Geometry check sheet. Reference: the model listing, model coordinates, mm. A direction names the side the tool comes from. Round coordinates to 2 decimals unless told otherwise and drop trailing zeros. Order: outer loops, then holes, each group sorted by start corner. A loop starts at its lowest first (then second) coordinate and runs counter-clockwise, first axis right, second up.
(1) Cross-section at C-C on x = -1.75. Enter the section's corners in (y, z), and give its area (3 significant figures).
(2) Set-up check for faces 1 (the face through (0, 3, 0)), 2 (the face through (-2, -2, 9.6)), 3 (the face through (0, -2.4, 4)): record each of +Z, -Z, +X, -X, +Y, -Y from which the full face is reachable in a straight line by a thin tool's end or side.
(3) Cross-section at A-A on y = 0. Enter the section's corners in (x, z), and give its area (3 significant figures).
(4) Cross-section at D-D on z = 9.75. Enter the section's corners in (x, y), and give its area (3 significant figures).
(5) Draft check along Y on faces 4 (the face through (0, 0, 11.2)), 5 (the face through (0, -4, 5)), 6 (the face through (-2.4, 0, 4)). Enter one of: pulls with the +Y half, pulls with the -Y half, needs draft (parallel to the pull), parting line crosses it, or undercut.
(6) Cross-section at B-B on z = 6.5. Enter the section's corners in (x, y), and give its area (3 significant figures).
(7) Thickness scan on L1, parallel to X at y = -1, z = 2.25; L2, parallel to Z at x = -0.25, y = 0. Record the ranges inside material, lowest first.
from build123d import *

# Parameters (mm, degrees)
F0_W     = 8
F0_H     = 8
F1_DEPTH = 9.6
F2_W     = 4.8
F2_H     = 4.8
F3_DEPTH = 8
F4_R     = 2.4
F5_DEPTH = 1.6


with BuildPart() as f1:
    # F0 (on Top) → F1 (new body)
    with BuildSketch(Plane.XY):
        Rectangle(F0_W, F0_H)
    extrude(amount=F1_DEPTH)

    # F2 (on face) → F3 (cut)
    with BuildSketch(Plane(origin=(0, 0, 0), x_dir=(1, 0, 0), z_dir=(0, 0, -1))):
        Rectangle(F2_W, F2_H)
    extrude(amount=-F3_DEPTH, mode=Mode.SUBTRACT)

    # F4 (on face) → F5 (join)
    with BuildSketch(Plane.XY.offset(9.6)):
        Circle(F4_R)
    extrude(amount=F5_DEPTH)


solid = f1.part
Found:
1. outline: (-4, 0) - (-2.4, 0) - (-2.4, 8) - (2.4, 8) - (2.4, 0) - (4, 0) - (4, 9.6) - (1.64, 9.6) - (1.64, 11.2) - (-1.64, 11.2) - (-1.64, 9.6) - (-4, 9.6) - close
1. area: 43.7 mm2
2. face 1: -Z, +X, -X, +Y, -Y
2. face 2: +Z
2. face 3: -Z
3. outline: (-4, 0) - (-2.4, 0) - (-2.4, 8) - (2.4, 8) - (2.4, 0) - (4, 0) - (4, 9.6) - (2.4, 9.6) - (2.4, 11.2) - (-2.4, 11.2) - (-2.4, 9.6) - (-4, 9.6) - close
3. area: 46.1 mm2
4. outline: circle Ø4.8 at (0, 0)
4. area: 18.1 mm2
5. face 4: needs draft
5. face 5: pulls with the -Y half
5. face 6: undercut
6. outline: (-4, -4) - (4, -4) - (4, 4) - (-4, 4) - close; hole (-2.4, -2.4) - (2.4, -2.4) - (2.4, 2.4) - (-2.4, 2.4) - close
6. area: 41.0 mm2
7. L1: x = -4 to -2.4, 2.4 to 4
7. L2: z = 8 to 11.2
